Geometry: final body of the model. Coordinates: model frame, mm. A direction names the side the tool comes from. Coordinates: 2 decimals unless noted, no trailing zeros. Order: outer loops, then holes, each group sorted by start corner. A loop starts at its lowest first (then second) coordinate and runs counter-clockwise, first axis right, second up. Notation, with made-up numbers: M -28,24 L 9,24 A28 ccw 9,45 Z; hole C -16,28 d8. An arc over 180 degrees is marked long. Write item = value, one per line.
from build123d import *

# Parameters (mm, degrees)
SKETCH1_W          = 120
SKETCH1_H          = 80
FRAME_DEPTH        = 4
SKETCH3_R          = 2
CUT_EXTRUDE1_DEPTH = 4
CRVPATTERN2_COUNT  = 10
CRVPATTERN2_PITCH  = 14.666666667
CRVPATTERN3_COUNT  = 8
CRVPATTERN3_PITCH  = 13.142857143
SKETCH4_R          = 2
CUT_EXTRUDE2_DEPTH = 4
CRVPATTERN5_COUNT  = 10
CRVPATTERN5_PITCH  = 14.666666667
CRVPATTERN6_COUNT  = 8
CRVPATTERN6_PITCH  = 13.142857143
SKETCH12_R         = 3
CUT_EXTRUDE4_DEPTH = 10


with BuildPart() as part:
    # Sketch1 → Frame (new body)
    with BuildSketch(Plane.XY):
        with BuildLine():
            Line((0, -12), (120, -12))
            ThreePointArc((120, -12), (140.485281374, -20.485281374), (132, 0))
            Line((132, 0), (132, 80))
            ThreePointArc((132, 80), (140.485281374, 100.485281374), (120, 92))
            Line((120, 92), (0, 92))
            ThreePointArc((0, 92), (-20.485281374, 100.485281374), (-12, 80))
            Line((-12, 80), (-12, 0))
            ThreePointArc((-12, 0), (-20.485281374, -20.485281374), (0, -12))
        make_face()
        with Locations((60, 40)):
            Rectangle(SKETCH1_W, SKETCH1_H, mode=Mode.SUBTRACT)
    extrude(amount=FRAME_DEPTH)

    # Sketch3 → Cut-Extrude1 (cut)
    with BuildSketch(Plane(origin=(0, 0, 0), x_dir=(-1, 0, 0), z_dir=(0, 0, -1))):
        with Locations((-126, 86)):
            Circle(SKETCH3_R)
    cut_extrude1 = extrude(amount=-CUT_EXTRUDE1_DEPTH, mode=Mode.SUBTRACT)

    # CrvPattern2: Cut-Extrude1 ×10, 1 skipped
    with Locations(*[(-i * CRVPATTERN2_PITCH, 0, 0) for i in range(1, CRVPATTERN2_COUNT) if i not in (9,)]):
        add(cut_extrude1, mode=Mode.SUBTRACT)

    # CrvPattern3: Cut-Extrude1 ×8, 1 skipped
    with Locations(*[(0, -i * CRVPATTERN3_PITCH, 0) for i in range(1, CRVPATTERN3_COUNT) if i not in (7,)]):
        add(cut_extrude1, mode=Mode.SUBTRACT)

    # Sketch4 → Cut-Extrude2 (cut)
    with BuildSketch(Plane(origin=(0, 0, 0), x_dir=(-1, 0, 0), z_dir=(0, 0, -1))):
        with Locations((6, -6)):
            Circle(SKETCH4_R)
    cut_extrude2 = extrude(amount=-CUT_EXTRUDE2_DEPTH, mode=Mode.SUBTRACT)

    # CrvPattern5: Cut-Extrude2 ×10
    with Locations(*[(i * CRVPATTERN5_PITCH, 0, 0) for i in range(1, CRVPATTERN5_COUNT)]):
        add(cut_extrude2, mode=Mode.SUBTRACT)

    # CrvPattern6: Cut-Extrude2 ×8
    with Locations(*[(0, i * CRVPATTERN6_PITCH, 0) for i in range(1, CRVPATTERN6_COUNT)]):
        add(cut_extrude2, mode=Mode.SUBTRACT)

    # Sketch12 → Cut-Extrude4 (cut)
    with BuildSketch(Plane(origin=(0, 0, 0), x_dir=(-1, 0, 0), z_dir=(0, 0, -1))):
        with Locations((-132, 92)):
            Circle(SKETCH12_R)
        with Locations((12, 92)):
            Circle(SKETCH12_R)
        with Locations((12, -12)):
            Circle(SKETCH12_R)
        with Locations((-132, -12)):
            Circle(SKETCH12_R)
    extrude(amount=-CUT_EXTRUDE4_DEPTH, mode=Mode.SUBTRACT)


solid = part.part
1) Section C-C, the plane z = 2.15. Give the number of separate pieces and of enclosed holes in the cut face, and give its area (3 significant figures).
Numbers:
separate_pieces = 1
enclosed_holes = 37
area = 6,220 mm²
2) Set-up query: faces 1 (the face through (61, 92, 2)), 2 (the face through (0, 39, 2)). Return all of +Z, -Z, +X, -X, +Y, -Y with unobstructed straight access to the full face (end or side cutting, diameter ignored); none if empty.
Numbers:
face_1 = +Z, -Z, +Y
face_2 = +Z, -Z
3) Mould query, pull axis X, two halves, no side actions, for faces 3 (the face through (132, 39, 2)), 4 (the face through (126.434, 70.905, 1.972)), 5 (the face through (50.76, -5.4, 1.97)), 6 (the face through (60, -2, 0)). Classes: pulls with the +X half, pulls with the -X half, needs draft (parallel to the pull), parting line crosses it, or undercut.
Numbers:
face_3 = pulls with the +X half
face_4 = undercut
face_5 = undercut
face_6 = needs draft
4) Line query: L1, parallel to X at y = 7.5, z = 3.8; L2, parallel to Y at x = 93, z = 3.85; L3, parallel to X at y = 13.5, z = 3.1. Output: solid intervals per line, ascending.
Numbers:
L1 = -12 to -7.97, -4.03 to 0, 120 to 124.03, 127.97 to 132
L2 = -12 to 0, 80 to 92
L3 = -12 to 0, 120 to 132
5) Pin query (flat end, axial travel): pin 1 (3.5 mm diameter, centred on x = 52.67, y = -6, fed in from -Z); pin 2 (1.2 mm diameter, centred on y = 53, z = 1.5, fed in from -X); pin 3 (1.5 mm diameter, centred on x = 106, z = 3, fed in from -Y); pin 4 (1 mm diameter, centred on x = 54, z = 2, fed in from +Y). Return the tip coordinate at first contact, or that it passes through.
Numbers:
pin_1 = through
pin_2 = -12
pin_3 = -12
pin_4 = 92
6) Section B-B, the plane y = 54. Return loops of the section in (x, z), and give its area (3 significant figures).
Numbers:
outline = M -12,0 L 0,0 L 0,4 L -12,4 Z; M 120,0 L 132,0 L 132,4 L 120,4 Z
area = 96.0 mm²
7) Section A-A, the plane x = 82. Return loops of the section in (y, z).
Numbers:
outline = M -12,0 L -8,0 L -8,4 L -12,4 Z; M -4,0 L 0,0 L 0,4 L -4,4 Z; M 80,0 L 84,0 L 84,4 L 80,4 Z; M 88,0 L 92,0 L 92,4 L 88,4 Z
